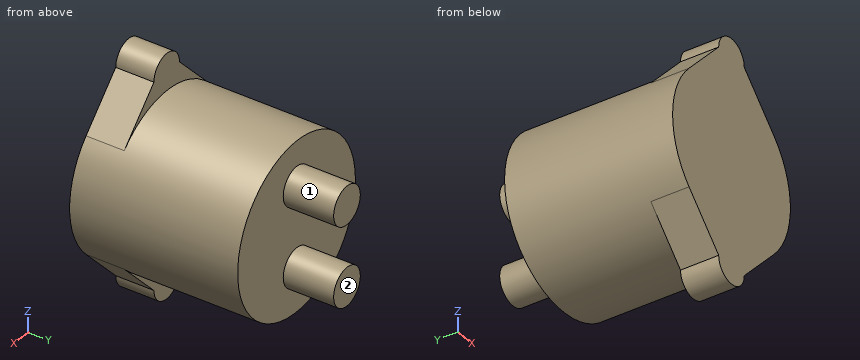
Autodesk Inventor part; units mm, degrees
ref_plane "YZ Plane" through (0, 0, 0) normal (1, 0, 0) x (0, 1, 0)
ref_plane "XZ Plane" through (0, 0, 0) normal (0, 1, 0) x (-1, 0, 0)
ref_plane "XY Plane" through (0, 0, 0) normal (0, 0, 1) x (1, 0, 0)
sketch "Sketch1" plane through (0, 0, 0) normal (0, 1, 0) x (-1, 0, 0)
  circle A0 centre (0, 0) radius 28.067
  dimension "d0" = 56.134
extrude "Extrusion1" add sketch "Sketch1" along normal blind 55.88
sketch "Sketch2" plane through (0, 55.88, 0) normal (0, 1, 0) x (1, 0, 0)
  circle A0 centre (0, -13.335) radius 6.35
  circle A1 centre (0, 13.335) radius 6.35
  point P0 (0, 0)
  dimension "d5" = 12.7
  dimension "d6" = 12.7
extrude "Extrusion2" add sketch "Sketch2" along normal blind 16.764
sketch "Sketch3" plane through (0, 0, 0) normal (0, -1, 0) x (1, 0, 0)
  circle A0 centre (0, 0) radius 28.067
  circle A1 centre (0, 34.163) radius 6.096
  circle A2 centre (0, -34.163) radius 6.096
  line L0 (6.096, 34.163) -> (20.2372, 19.4477)
  line L1 (6.096, -34.163) -> (20.2372, -19.4477)
  line L2 (-6.096, 34.163) -> (-20.2372, 19.4477)
  line L3 (-6.096, -34.163) -> (-20.2372, -19.4477)
extrude "Extrusion3" add sketch "Sketch3" against normal blind 12.7 contours A0 A1 L0 | A0 L2 A1 | A1
sketch "Sketch4" plane through (0, 0, 0) normal (0, -1, 0) x (1, 0, 0)
  circle A0 centre (0, 0) radius 28.067
  circle A1 centre (0, -34.163) radius 6.096
  line L0 (6.096, -34.163) -> (20.2372, -19.4477)
  line L1 (-6.096, -34.163) -> (-20.2372, -19.4477)
extrude "Extrusion4" add sketch "Sketch4" against normal blind 12.7
properties part number "Precharge_Relay"
Part model, mm, in its own coordinate system. Face numbers are marked on the shaded views. A direction names the side the tool comes from. Coordinates: 2 decimals unless noted, no trailing zeros. Loops run counter-clockwise (first coordinate to the right, second up) from the corner with the lowest first, then second, coordinate; pieces in that order, holes last. Notation, with made-up numbers: M -26,88 L 5,88 A20 ccw 5,124 Z; hole C 25.5,-36.75 d3. An arc over 180 degrees is marked long. Use a Markdown table: item, result. Add a question column.
Q1. Which spindle directions (+Z, -Z, +X, -X, +Y, -Y) get a long thin tool onto all of the face, cutting with end or side? Do the marked faces 1 and 2. Say none if no direction does.
Q2. Cut at A-A (x = 0). Write the cut outline in (y, z) (3 decimals).
Q3. Pin check, flat tips, straight feed: P1, Ø6, axis at y = 64, z = -12.5, coming from the +X side; P2, Ø3, axis at x = 13, y = 49.5, coming from the -Z side; P3, Ø1, axis at x = 12.5, y = 45, coming from the +Z side. Stop position of each tip, or through.
Q4. Cut at B-B (z = 0). Write the cut outline in (x, y).
Q5. Probe L1, parallel to Y at x = -23, z = -15; L2, parallel to Z at x = 4, y = 64; L3, parallel to X at y = 32, z = 14. List the from-to ranges inside material, lowest first.
Q6. Cut at C-C (y = 37). Write the cut outline in (x, z).
Q7. Cut at D-D (x = 7.5). Write the cut outline in (y, z), and give its area (3 significant figures).
Worked out:
| question | item | result |
|---|---|---|
| 1 | face 1 | +Y |
| 1 | face 2 | +Z, -Z, +X, -X, +Y |
| 2 | outline | M 0,-40.259 L 12.7,-40.259 L 12.7,-28.067 L 55.88,-28.067 L 55.88,-19.685 L 72.644,-19.685 L 72.644,-6.985 L 55.88,-6.985 L 55.88,6.985 L 72.644,6.985 L 72.644,19.685 L 55.88,19.685 L 55.88,28.067 L 12.7,28.067 L 12.7,40.259 L 0,40.259 Z |
| 3 | P1 | stops at x = 6.35 |
| 3 | P2 | stops at z = -25.6 |
| 3 | P3 | stops at z = 25.37 |
| 4 | outline | M -28.07,0 L 28.07,0 L 28.07,55.88 L -28.07,55.88 Z |
| 5 | L1 | y = 0 to 55.88 |
| 5 | L2 | z = -18.27 to -8.4, 8.4 to 18.27 |
| 5 | L3 | x = -24.33 to 24.33 |
| 6 | outline | C 0,0 d56.13 |
| 7 | outline | M 0,-32.7 L 12.7,-32.7 L 12.7,-27.05 L 55.88,-27.05 L 55.88,27.05 L 12.7,27.05 L 12.7,32.7 L 0,32.7 Z |
| 7 | area | 3,170 mm2 |
